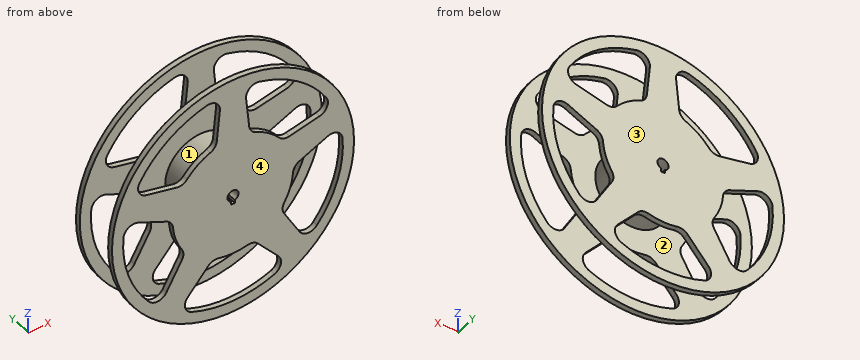
```python
from build123d import *

# Parameters (mm, degrees)
CUT_EXTRUDE1_DEPTH = 128.2030377
CIRPATTERN1_COUNT  = 5
CUT_EXTRUDE2_DEPTH = 128.2030377


with BuildPart() as part:
    # Sketch1 → Revolve1 (revolve)
    with BuildSketch(Plane.XY, mode=Mode.PRIVATE) as revolve1_sk:
        Polygon((0, 0), (86.36, 0), (86.36, 3.78), (25.4, 3.78), (25.4, 31.78), (86.36, 31.78), (86.36, 35.56), (0, 35.56), align=None)
    revolve(revolve1_sk.sketch.rotate(Axis((0, 35.56, 0), (0, -1, 0)), 180), axis=Axis((0, 35.56, 0), (0, -1, 0)))

    # Sketch2 → Cut-Extrude1 (cut, through all)
    with BuildSketch(Plane(origin=(0, 35.56, 0), x_dir=(1, 0, 0), z_dir=(0, 1, 0))):
        with BuildLine():
            Line((-32.38324098, 60.461396247), (-17.736798391, 44.055966634))
            ThreePointArc((-17.736798391, 44.055966634), (-14.309566496, 41.852699526), (-10.237061566, 41.730192332))
            ThreePointArc((-10.237061566, 41.730192332), (0, 42.967503786), (10.237061566, 41.730192332))
            ThreePointArc((10.237061566, 41.730192332), (14.309566496, 41.852699526), (17.736798391, 44.055966634))
            Line((17.736798391, 44.055966634), (32.38324098, 60.461396247))
            ThreePointArc((32.38324098, 60.461396247), (34.12253228, 67.255277706), (29.573893077, 72.593052609))
            ThreePointArc((29.573893077, 72.593052609), (0, 78.386009204), (-29.573893077, 72.593052609))
            ThreePointArc((-29.573893077, 72.593052609), (-34.12253228, 67.255277706), (-32.38324098, 60.461396247))
        make_face()
    cut_extrude1 = extrude(amount=-CUT_EXTRUDE1_DEPTH, mode=Mode.SUBTRACT)

    # CirPattern1: Cut-Extrude1 ×5 about axis
    cirpattern1_axis = Axis((0, 0, 0), (0, 1, 0))
    for i in range(1, CIRPATTERN1_COUNT):
        add(cut_extrude1.rotate(cirpattern1_axis, i * 360 / CIRPATTERN1_COUNT), mode=Mode.SUBTRACT)

    # Sketch3 → Cut-Extrude2 (cut, through all)
    with BuildSketch(Plane(origin=(0, 35.56, 0), x_dir=(1, 0, 0), z_dir=(0, 1, 0))):
        with BuildLine():
            Line((-1.2891518, 3.753540222), (-1.2891518, 6.049382139))
            Line((-1.2891518, 6.049382139), (1.2891518, 6.049382139))
            Line((1.2891518, 6.049382139), (1.2891518, 3.753540222))
            ThreePointArc((1.2891518, 3.753540222), (0, -3.96875), (-1.2891518, 3.753540222))
        make_face()
    extrude(amount=-CUT_EXTRUDE2_DEPTH, mode=Mode.SUBTRACT)


solid = part.part
```
The model under review builds one solid part; all positions refer to its coordinate system, in mm. Face numbers are marked on the shaded views. Give positions to 0.01 mm unless a question says otherwise; leave off trailing zeros. Write each loop counter-clockwise with the first axis right and the second up, starting at its lowest first coordinate (ties: lowest second). Pieces come first, ordered by that corner, then holes. Notation, with made-up numbers: M 25.25,-1 L 45.25,-1 A23 ccw 45.25,34 Z; hole C 18.25,42.5 d6. An arc over 180 degrees is marked long. Answer in a Markdown table with one row per item.
Item 1: For P1, Ø5, axis at y = 15.5, z = 15, coming from the -X side; P2, Ø2, axis at x = 55, z = 23.5, coming from the -Y side; P3, Ø0.8, axis at x = 0, y = 17.5, coming from the +Z side; P4, Ø0.7, axis at y = 13.5, z = -4.5, coming from the +X side, all flat-tipped, find the tip position at first contact; note any pin that passes through.
Check sheet entries:
| item | result |
|---|---|
| P1 | x = -22.11 |
| P2 | y = 0 |
| P3 | z = 25.4 |
| P4 | x = 25.06 |
Item 2: Draft analysis for pull direction Y (two halves, no side actions). For the marked faces 1, 2, 3 and 4, state which applies: +Y half, -Y half, draft (parallel to the pull), parting line (faces both ways), or undercut.
Check sheet entries:
| item | result |
|---|---|
| face 1 | undercut |
| face 2 | undercut |
| face 3 | +Y half |
| face 4 | -Y half |
Item 3: For line 1 along Y through (x, z) = (31, -40); line 2 along Z through (x, y) = (0, 27.5); line 3 along Z through (x, y) = (21, 2.5), list the stretches that pass through material, from the lowest coordinate up.
Check sheet entries:
| item | result |
|---|---|
| line 1 | 0 to 3.78, 31.78 to 35.56 |
| line 2 | -25.4 to -6.05, 3.97 to 25.4 |
| line 3 | -83.77 to -75.52, -47.71 to 37.49, 75.52 to 83.77 |
Item 4: Add section A-A on z = 0. State how many separate pieces and enclosed holes the cut face has, plus the area to 3 significant figures.
Check sheet entries:
| item | result |
|---|---|
| separate pieces | 6 |
| enclosed holes | 0 |
| area | 1,920 mm2 |
Item 5: Add section B-B on y = 23.5. Give the boundary of the cut face in (x, z).
Check sheet entries:
| item | result |
|---|---|
| outline | C 0,0 d50.8; hole M -1.29,-6.05 L 1.29,-6.05 L 1.29,-3.75 A3.97 ccw long -1.29,-3.75 Z |
Item 6: Add section C-C on x = 57. Give the boundary of the cut face in (y, z), plus the area to 3 significant figures.
Check sheet entries:
| item | result |
|---|---|
| outline | M 0,-64.88 L 3.78,-64.88 L 3.78,-52.68 L 0,-52.68 Z; M 0,7.49 L 3.78,7.49 L 3.78,28.85 L 0,28.85 Z; M 0,53.81 L 3.78,53.81 L 3.78,64.88 L 0,64.88 Z; M 31.78,-64.88 L 35.56,-64.88 L 35.56,-52.68 L 31.78,-52.68 Z; M 31.78,7.49 L 35.56,7.49 L 35.56,28.85 L 31.78,28.85 Z; M 31.78,53.81 L 35.56,53.81 L 35.56,64.88 L 31.78,64.88 Z |
| area | 337 mm2 |
